The drawing under review shows one solid part. Ordinate dimensions are in mm from its lowest x, y, z. Round coordinates to 2 decimals unless told otherwise and drop trailing zeros. Write each loop counter-clockwise with the first axis right and the second up, starting at its lowest first coordinate (ties: lowest second). Pieces come first, ordered by that corner, then holes. Notation, with made-up numbers: (56, 11) -> (101, 11) arc R23 ccw to (101, 27) -> close; hole circle Ø10 at (-23.75, 60.5). An arc over 180 degrees is marked (long way). Use CSV: the item, a comma, the result in double quotes. Start each with the question number.
1) Take a section at C-C, the plane x = 62.5. Give the boundary of the cut face in (y, z).
2) For pin 1 Ø1.5 at (x, y) = (92, 4) entering from -Z; pin 2 Ø6 at (x, z) = (74.5, 40) entering from -Y; pin 3 Ø0.9 at (y, z) = (1.5, 71) entering from +X; pin 4 Ø2.5 at (x, z) = (39, 38.29) entering from +Y, all flat-tipped, find the tip position at first contact; note any pin that passes through.
3) Wall thickness on probe 1 along X at (y, z) = (4.5, 15.5) (1 decimal); probe 2 along X at (y, z) = (1.85, 73.5); probe 3 along Y at (x, z) = (33, 109): over which ranges is each line inside the solid? List them lowest first. Write a range as [from, to].
4) Take a section at A-A, the plane x = 39. Give the boundary of the cut face in (y, z).
5) Take a section at B-B, the plane z = 34.5. Give the boundary of the cut face in (x, y), then the cut area to 3 significant figures.
6) Take a section at D-D, the plane y = 4.3. State how many separate pieces and enclosed holes the cut face has, then the cut area to 4 significant figures.
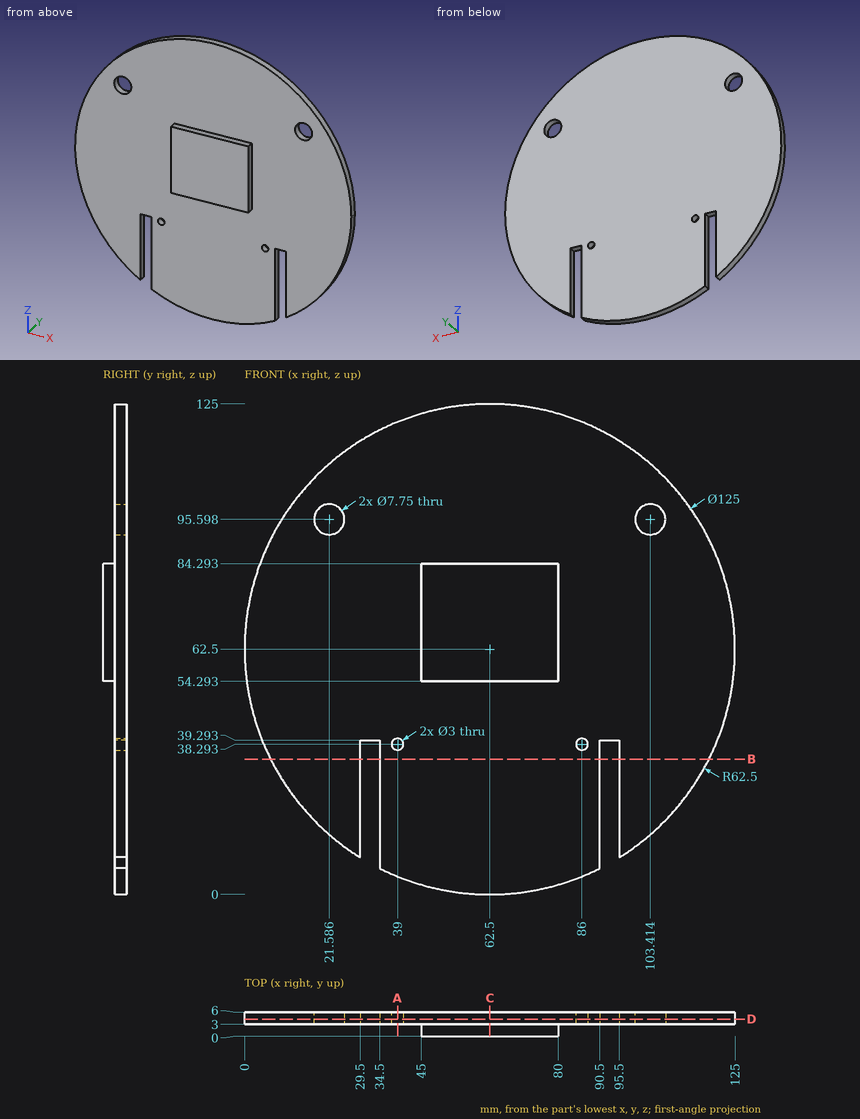
Values found:
1,outline,"(0, 54.29) -> (3, 54.29) -> (3, 0) -> (6, 0) -> (6, 125) -> (3, 125) -> (3, 84.29) -> (0, 84.29) -> close"
2,pin 1,"z = 39.29"
2,pin 2,"y = 3"
2,pin 3,"x = 80"
2,pin 4,"through"
3,probe 1,"[21.3, 29.5], [34.5, 90.5], [95.5, 103.7]"
3,probe 2,"[45, 80]"
3,probe 3,"[3, 6]"
4,outline,"(3, 4.59) -> (6, 4.59) -> (6, 36.79) -> (3, 36.79) -> close; (3, 39.79) -> (6, 39.79) -> (6, 120.41) -> (3, 120.41) -> close"
5,outline,"(6.62, 3) -> (29.5, 3) -> (29.5, 6) -> (6.62, 6) -> close; (34.5, 3) -> (90.5, 3) -> (90.5, 6) -> (34.5, 6) -> close; (95.5, 3) -> (118.38, 3) -> (118.38, 6) -> (95.5, 6) -> close"
5,area,"305 mm²"
6,separate pieces,"1"
6,enclosed holes,"4"
6,area,"11,850 mm²"
